Autodesk Inventor part; units mm, degrees
ref_plane "YZ Plane" through (0, 0, 0) normal (1, 0, 0) x (0, 1, 0)
ref_plane "XZ Plane" through (0, 0, 0) normal (0, 1, 0) x (-1, 0, 0)
ref_plane "XY Plane" through (0, 0, 0) normal (0, 0, 1) x (1, 0, 0)
sketch "Sketch1" plane through (0, 0, 0) normal (1, 0, 0) x (0, 1, 0)
  circle A0 centre (0, 0) radius 3.5
  circle A1 centre (0, 0) radius 1.25
  line L0 (0, -3.5) -> (0.5, -3.5)
  line L1 (0.5, -3.5) -> (0.5, -13.5)
  line L2 (0.5, -13.5) -> (0, -13.5)
  line L3 (0, -13.5) -> (0, -3.5)
  line L4 (0.5, -13.5) -> (2.0279, -13.5)
  line L5 (2.0279, -13.5) -> (2.0279, -5.25)
  line L6 (2.0279, -5.25) -> (0.5, -5.25)
  line L7 (0.5, -5.25) -> (0.5, -13.5)
  line L8 (0, -3.5) -> (-0.5, -3.5)
  line L9 (-0.5, -3.5) -> (-0.5, -13.5)
  line L10 (-0.5, -13.5) -> (0, -13.5)
  line L11 (-0.5, -13.5) -> (-2.0279, -13.5)
  line L12 (-2.0279, -13.5) -> (-2.0279, -5.25)
  line L13 (-2.0279, -5.25) -> (-0.5, -5.25)
  line L14 (-0.5, -5.25) -> (-0.5, -13.5)
  line L15 (-0.5, -13.5) -> (-2.0279, -13.5)
  line L16 (-2.0279, -13.5) -> (-2.0279, -2.6024)
  line L17 (-2.0279, -2.6024) -> (-0.5, -2.6024)
  line L18 (-0.5, -2.6024) -> (-0.5, -13.5)
  line L19 (2.0279, -13.5) -> (0.5, -13.5)
  line L20 (0.5, -13.5) -> (0.5, -2.6024)
  line L21 (0.5, -2.6024) -> (2.0279, -2.6024)
  line L22 (2.0279, -2.6024) -> (2.0279, -13.5)
  dimension "d0" = 7
  dimension "d1" = 2.5
  dimension "d2" = 0.5
  dimension "d3" = 10
extrude "Extrusion1" add sketch "Sketch1" along normal blind 5 contours A0 L22 L21 L20 L18 L17 L16 | L16 L17 L18 A0 | A0 L18 L9 L13 L16 | L22 L6 L1 L20 A0 | A0 L20 L21 L22 | L13 L9 L11 L12 | L5 L4 L1 L6
sketch "Sketch3" plane through (0, 2.0279, -2.8527) normal (0, 1, 0) x (1, 0, 0)
  line L0 (0, 0) -> (5.024, 10.7024)
  circle A0 centre (2.512, 5.3512) radius 0.9732
  point P0 (0, -2.8527)
extrude "Extrusion3" cut sketch "Sketch3" against normal blind 10
properties part number "servo attachment"
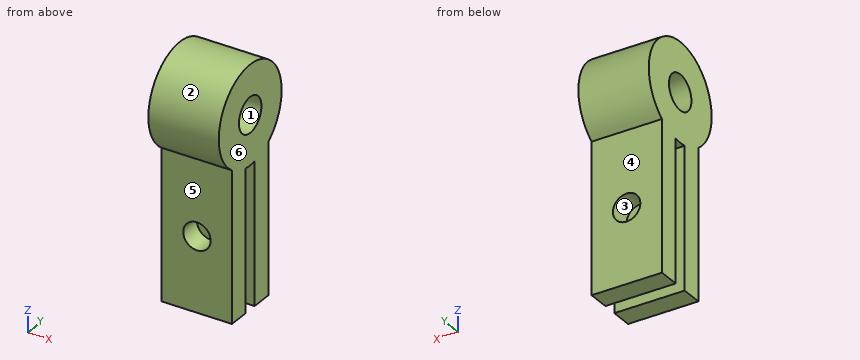
The listing builds one solid part. Answer for the finished solid, in the listing's coordinates (mm). Face numbers are marked on the shaded views. A direction names the side the tool comes from. Give positions to 0.01 mm unless a question says otherwise; leave off trailing zeros. Write each loop counter-clockwise with the first axis right and the second up, starting at its lowest first coordinate (ties: lowest second). Pieces come first, ordered by that corner, then holes. Notation, with made-up numbers: (88, 70) -> (132, 70) arc R19 cw to (132, 104) -> close; hole circle Ø5 at (-32.75, -1). An arc over 180 degrees is marked (long way). One line per question, with ' | ' between items. Start each with the question number.
1. Section B-B (x = 4.5) is taken. Determine the outline of the cut face in (y, z).
2. Section A-A (z = -12.25) is taken. Determine the outline of the cut face in (x, y), plus the area to 3 significant figures.
3. Given pin 1 Ø2.5 at (x, z) = (3.5, -10.5) entering from -Y; pin 2 Ø2.5 at (x, z) = (3, -11) entering from +Y, each flat-ended and moving along its own axis, determine where each tip first touches the part or whether it passes through.
4. Section C-C (y = -1) is taken. Determine the outline of the cut face in (x, z).
5. Section D-D (x = 2.2) is taken. Determine the outline of the cut face in (y, z), plus the area to 3 significant figures.
6. Find the intervals of material crossed by probe 1 along Z at (x, y) = (2.9, 0); probe 2 along Z at (x, y) = (2.1, -1); probe 3 along Y at (x, z) = (2.45, -9.5), in increasing order.
7. For the marked faces 5 and 6, determine the directions among +Z, -Z, +X, -X, +Y, -Y from which every point of the face is accessible in a straight line to the end or side of a thin tool.
8. For a pull along Z with two mould halves and no side action, classify the marked faces 1, 2, 3 and 4 as pulls with the +Z half, pulls with the -Z half, needs draft (parallel to the pull), parting line crosses it, or undercut.
Response values:
1) outline: (-2.03, -13.5) -> (-0.5, -13.5) -> (-0.5, -3.46) arc R3.5 ccw to (0.5, -3.46) -> (0.5, -13.5) -> (2.03, -13.5) -> (2.03, -2.85) arc R3.5 ccw (long way) to (-2.03, -2.85) -> close; hole circle Ø2.5 at (0, 0)
2) outline: (0, -2.03) -> (5, -2.03) -> (5, -0.5) -> (0, -0.5) -> close; (0, 0.5) -> (5, 0.5) -> (5, 2.03) -> (0, 2.03) -> close | area: 15.3 mm2
3) pin 1: y = -2.03 | pin 2: y = 2.03
4) outline: (0, -13.5) -> (5, -13.5) -> (5, -0.75) -> (0, -0.75) -> close; (0, 0.75) -> (5, 0.75) -> (5, 3.35) -> (0, 3.35) -> close; hole circle Ø1.95 at (2.51, -8.2)
5) outline: (-2.03, -13.5) -> (-0.5, -13.5) -> (-0.5, -9.13) -> (-2.03, -9.13) -> close; (-2.03, -7.28) -> (-0.5, -7.28) -> (-0.5, -3.46) arc R3.5 ccw to (0.5, -3.46) -> (0.5, -7.28) -> (2.03, -7.28) -> (2.03, -2.85) arc R3.5 ccw (long way) to (-2.03, -2.85) -> close; (0.5, -13.5) -> (2.03, -13.5) -> (2.03, -9.13) -> (0.5, -9.13) -> close; hole circle Ø2.5 at (0, 0) | area: 59.3 mm2
6) probe 1: -3.5 to -1.25, 1.25 to 3.5 | probe 2: -13.5 to -9.09, -7.32 to -0.75, 0.75 to 3.35 | probe 3: -2.03 to -0.5, 0.5 to 2.03
7) face 5: -Z, +X, -X, -Y | face 6: +Z, -Z, +X, +Y, -Y
8) face 1: undercut | face 2: parting line crosses it | face 3: undercut | face 4: needs draft
